Geometry: see drawing. Coordinates: mm, zero at the bounding-box minimum. A direction names the side the tool comes from. Round coordinates to 2 decimals unless told otherwise and drop trailing zeros. Write each loop counter-clockwise with the first axis right and the second up, starting at its lowest first coordinate (ties: lowest second). Pieces come first, ordered by that corner, then holes.
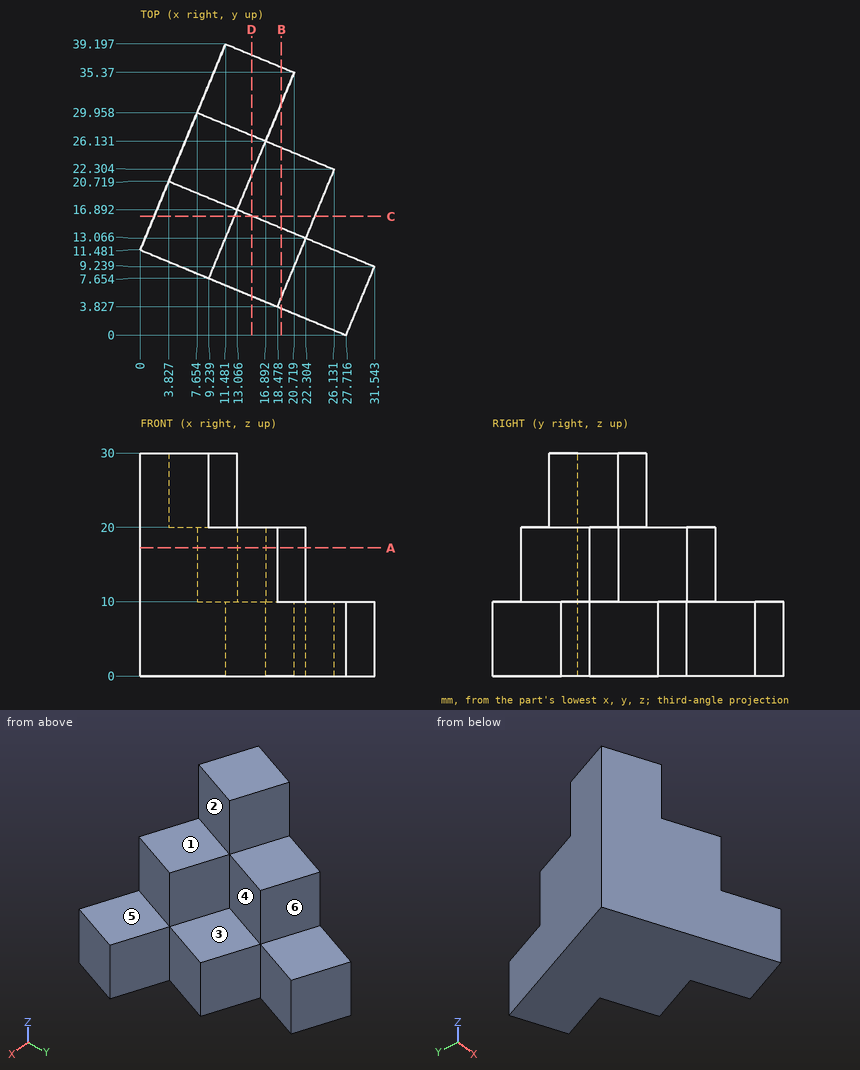
1) Section query D-D on x = 15. Return the cut outline in (y, z) (1 decimal).
Taken from the geometry:
outline: (5.3, 0) - (37.7, 0) - (37.7, 10) - (26.9, 10) - (26.9, 20) - (21.6, 20) - (21.6, 10) - (16.1, 10) - (16.1, 20) - (5.3, 20) - close
2) Section query B-B on x = 19. Return the cut outline in (y, z) (1 decimal).
Taken from the geometry:
outline: (3.6, 0) - (25.3, 0) - (25.3, 10) - (14.4, 10) - (14.4, 20) - (5.1, 20) - (5.1, 10) - (3.6, 10) - close; (31.2, 0) - (36.1, 0) - (36.1, 10) - (31.2, 10) - close
3) Section query A-A on z = 17.25. Return the cut outline in (x, y) (1 decimal), then the cut area to 3 significant figures.
Taken from the geometry:
outline: (0, 11.5) - (18.5, 3.8) - (22.3, 13.1) - (13.1, 16.9) - (16.9, 26.1) - (7.7, 30) - close
area: 300 mm2
4) Reachability of the marked faces 4, 5 and 6 from +Z, -Z, +X, -X, +Y, -Y: full face, straight path, thin tool, end or side. Return the list, or none.
Taken from the geometry:
face 4: +Z, +X
face 5: +Z, +X, -Y
face 6: +Z, +X, +Y
5) Section query C-C on y = 16. Return the cut outline in (x, z) (1 decimal).
Taken from the geometry:
outline: (1.9, 0) - (23.5, 0) - (23.5, 10) - (15.2, 10) - (15.2, 20) - (12.7, 20) - (12.7, 30) - (1.9, 30) - close
6) Contact query for flat-ended pins moving along their axis: P1, Ø3, axis at x = 19, z = 12.5, coming from the +Y side (1 decimal); P2, Ø12, axis at y = 33, z = 14.5, coming from the +X side; P3, Ø4, axis at x = 22, y = 9, coming from the +Z side. Output: stop coordinate, or through.
Taken from the geometry:
P1: stops at y = 15.1
P2: stops at x = 20.72
P3: stops at z = 20
7) Material intervals for line 1 (Z direction, x = 9, y = 20.5); line 2 (Z direction, x = 21, y = 4.5); line 3 (Y direction, x = 16.5, z = 9.5) (1 decimal), sorted ascending.
Taken from the geometry:
line 1: z = 0 to 20
line 2: z = 0 to 10
line 3: y = 4.6 to 37.1
8) Pull-direction query (Y, two-part tool) for the marked faces 1, 2 and 3; classes: released by +Y, released by -Y, zero draft, split by the parting line, or undercut.
Taken from the geometry:
face 1: zero draft
face 2: released by -Y
face 3: undercut
